```python
from build123d import *

# Parameters (mm, degrees)
F1_DEPTH = 25.4
F2_W     = 23.3461521566
F2_H     = 46.9620153308
F3_DEPTH = 17.78
F4_W     = 25.4
F4_H     = 7.1507450193
F4_W_2   = 26.6700030029
F5_DEPTH = 17.78
F4_H_2   = 6.5157404274
F6_DEPTH = 17.78
F7_W     = 22.2250013612
F7_H     = 14.2875015736
F8_DEPTH = 17.78


with BuildPart() as f1:
    # F0 (on Top) → F1 (new body)
    with BuildSketch(Plane.XY):
        with BuildLine():
            Line((26.0350015014, 37.782497704), (-26.0350015014, 37.782497704))
            Line((-26.0350015014, 37.782497704), (-26.0350015014, -37.782497704))
            Line((-26.0350015014, -37.782497704), (26.0350015014, -37.782497704))
            Line((26.0350015014, -37.782497704), (26.0350015014, -14.2516041014))
            ThreePointArc((26.0350015014, -14.2516041014), (11.7833974, 0), (26.0350015014, 14.2516041014))
            Line((26.0350015014, 14.2516041014), (26.0350015014, 37.782497704))
        make_face()
    extrude(amount=F1_DEPTH)

    # F2 (on face) → F3 (cut)
    with BuildSketch(Plane.XY.offset(25.4)):
        with Locations((-26.0350015014, 0)):
            Rectangle(F2_W, F2_H)
    extrude(amount=-F3_DEPTH, mode=Mode.SUBTRACT)

    # F4 (on face) → F5 (cut)
    with BuildSketch(Plane.XY.offset(25.4)):
        with Locations((-13.3350015014, -34.2071251944)):
            Rectangle(F4_W, F4_H)
        with Locations((12.7, -34.2071251944)):
            Rectangle(F4_W_2, F4_H)
    extrude(amount=-F5_DEPTH, mode=Mode.SUBTRACT)

    # F4 (on face) → F6 (cut)
    with BuildSketch(Plane.XY.offset(25.4)):
        with Locations((12.7, 34.5246274903)):
            Rectangle(F4_W_2, F4_H_2)
        with Locations((-13.3350015014, 34.5246274903)):
            Rectangle(F4_W, F4_H_2)
    extrude(amount=-F6_DEPTH, mode=Mode.SUBTRACT)

    # F7 (on face) → F8 (cut)
    with BuildSketch(Plane.XY.offset(25.4)):
        with Locations((14.9225008208, 23.9712502807)):
            Rectangle(F7_W, F7_H)
    extrude(amount=-F8_DEPTH, mode=Mode.SUBTRACT)


solid = f1.part
```
Check sheet for the modelled part. Datum: model origin and axes. Units: mm. A direction names the side the tool comes from. Give positions to 0.01 mm unless a question says otherwise; leave off trailing zeros. Order: outer loops, then holes, each group sorted by start corner. A loop starts at its lowest first (then second) coordinate and runs counter-clockwise, first axis right, second up. Notation, with made-up numbers: M 43,9.5 L 89,9.5 A17 ccw 89,33.5 Z; hole C 86.25,-38.75 d7. An arc over 180 degrees is marked long. Answer in a Markdown table with one row per item. Add a question column.
Q1. Gauge pin test, flat ends, axial feed: pin 1 Ø5.5 at (y, z) = (-2.5, 17) entering from -X; pin 2 Ø1.5 at (x, z) = (13.5, 15.5) entering from +Y; pin 3 Ø4.5 at (y, z) = (27, 12.5) entering from +X. Record the tip position at first contact, or that the pin passes through.
Q2. Thickness scan on L1, parallel to Y at x = -20, z = 14.25; L2, parallel to X at y = 21.5, z = 12; L3, parallel to X at y = 29, z = 20 (3 decimals). Record the ranges inside material, lowest first.
Q3. Sectioned sample at A-A, the plane x = -2. Record the boundary of the cut face in (y, z).
Q4. Sectioned sample at C-C, the plane y = 0. Record the boundary of the cut face in (x, z) (3 decimals), and give its area (3 significant figures).
Q5. Access from +Z, -Z, +X, -X, +Y, -Y to the whole of each face (thin tool, end or side, straight path). Record for faces 1 (the flat face through (0, -30.632, 17)), 2 (the flat face through (-20, 0, 7.62)), 3 (the flat face through (15, 24, 7.62)), 4 (the flat face through (0, 35, 7.62)).
Verdict:
| question | item | result |
|---|---|---|
| 1 | pin 1 | x = -14.36 |
| 1 | pin 2 | y = 31.27 |
| 1 | pin 3 | x = 3.81 |
| 2 | L1 | -30.63 to -23.48, 23.48 to 31.27 |
| 2 | L2 | -14.36 to 3.81 |
| 2 | L3 | -26.035 to 3.81 |
| 3 | outline | M -37.78,0 L 37.78,0 L 37.78,7.62 L 31.27,7.62 L 31.27,25.4 L -30.63,25.4 L -30.63,7.62 L -37.78,7.62 Z |
| 4 | outline | M -26.035,0 L 11.783,0 L 11.783,25.4 L -14.362,25.4 L -14.362,7.62 L -26.035,7.62 Z |
| 4 | area | 753 mm² |
| 5 | face 1 | +Z, +X, -X, -Y |
| 5 | face 2 | +Z, -X |
| 5 | face 3 | +Z, +X |
| 5 | face 4 | +Z, +X, -X, +Y |
